Autodesk Inventor part; units mm, degrees
ref_plane "YZ Plane" through (0, 0, 0) normal (1, 0, 0) x (0, 1, 0)
ref_plane "XZ Plane" through (0, 0, 0) normal (0, 1, 0) x (-1, 0, 0)
ref_plane "XY Plane" through (0, 0, 0) normal (0, 0, 1) x (1, 0, 0)
sketch "Sketch1" plane through (0, 0, 0) normal (0, 0, 1) x (1, 0, 0)
  line L0 (0, 0) -> (26.9875, 0)
  line L1 (26.9875, 5.08) -> (0, 5.08)
  line L2 (0, 5.08) -> (0, 0)
  arc A0 (26.9875, 4.1275) -> (26.9875, 0.9525) centre (26.9875, 2.54) ccw
  line L3 (26.9875, 0) -> (26.9875, 0.9525)
  line L4 (26.9875, 4.1275) -> (26.9875, 5.08)
  dimension "d0" = 5.08
  dimension "d1" = 26.9875
  dimension "d2" = 3.175
revolve "Revolution1" add sketch "Sketch1" angle 360 about axis through (0, 5.08, 0) along (0, -1, 0)
sketch "Sketch2" plane through (0, 5.08, 0) normal (0, 1, 0) x (1, 0, 0)
  line L0 (-22.0146, 3.0506) -> (-3.175, 3.1571)
  line L1 (3.175, 3.193) -> (21.9787, 3.2993)
  line L2 (-3.175, -21.997) -> (-3.175, -3.193)
  line L3 (-3.175, 3.1571) -> (-3.175, 21.997)
  arc A0 (-3.175, 21.997) -> (-22.0146, 3.0506) centre (0, 0) ccw
  line L4 (-21.9787, -3.2993) -> (-3.175, -3.193)
  line L5 (3.175, -3.1571) -> (22.0146, -3.0506)
  arc A1 (-21.9787, -3.2993) -> (-3.175, -21.997) centre (0, 0) ccw
  line L6 (3.175, -21.997) -> (3.175, -3.1571)
  line L7 (3.175, 3.193) -> (3.175, 21.997)
  arc A2 (3.175, -21.997) -> (22.0146, -3.0506) centre (0, 0) ccw
  arc A3 (21.9787, 3.2993) -> (3.175, 21.997) centre (0, 0) ccw
extrude "Extrusion1" cut sketch "Sketch2" against normal blind 25.4
sketch "Sketch3" plane through (0, 5.08, 0) normal (0, 1, 0) x (1, 0, 0)
  arc A0 (-1.0795, -0.9837) -> (-1.0795, 0.9837) centre (0, 0) ccw
  line L0 (-1.0795, -0.9837) -> (-1.0795, 0.9837)
  dimension "d11" = 2.921
  dimension "d12" = 1.0795
extrude "Extrusion2" cut sketch "Sketch3" against normal blind 25.4
fillet "Fillet1" radius 1.585 12 edges at (-3.175, 2.54, -3.1571) (3.175, 2.54, -3.193) (3.175, 2.54, 3.1571) (-3.175, 2.54, 3.193) (-21.9787, 2.54, 3.2993) (-3.175, 2.54, 21.997) (3.175, 2.54, 21.997) (22.0146, 2.54, 3.0506) (21.9787, 2.54, -3.2993) (3.175, 2.54, -21.997) (-3.175, 2.54, -21.997) (-22.0146, 2.54, -3.0506)
chamfer "Chamfer1" distance 1.585 angle 45 48 edges at (-12.4262, 5.08, -3.1048) (-21.348, 5.08, -3.6563) (-15.7598, 5.08, -15.671) (-3.7769, 5.08, -21.3269) (-3.175, 5.08, -12.4084) (-3.6361, 5.08, -3.6156) (-12.4172, 5.08, 3.2453) (-3.6424, 5.08, 3.6631) (-3.175, 5.08, 12.4353) (-3.7769, 5.08, 21.3269) (-15.671, 5.08, 15.7598) (-21.3052, 5.08, 3.8974) (12.4262, 5.08, 3.1048) (21.348, 5.08, 3.6563) (15.7598, 5.08, 15.671) (3.7769, 5.08, 21.3269) (3.175, 5.08, 12.4084) (3.6361, 5.08, 3.6156) (12.4172, 5.08, -3.2453) (3.6424, 5.08, -3.6631) (3.175, 5.08, -12.4353) (3.7769, 5.08, -21.3269) (15.671, 5.08, -15.7598) (21.3052, 5.08, -3.8974) (-3.6361, 0, -3.6156) (-12.4262, 0, -3.1048) (-21.348, 0, -3.6563) (-15.7598, 0, -15.671) (-3.7769, 0, -21.3269) (-3.175, 0, -12.4084) (-3.175, 0, 12.4353) (-3.6424, 0, 3.6631) (-12.4172, 0, 3.2453) (-21.3052, 0, 3.8974) (-15.671, 0, 15.7598) (-3.7769, 0, 21.3269) (3.175, 0, 12.4084) (3.7769, 0, 21.3269) (15.7598, 0, 15.671) (21.348, 0, 3.6563) (12.4262, 0, 3.1048) (3.6361, 0, 3.6156) (3.175, 0, -12.4353) (3.6424, 0, -3.6631) (12.4172, 0, -3.2453) (21.3052, 0, -3.8974) (15.671, 0, -15.7598) (3.7769, 0, -21.3269)
properties part number "Wheel"
CAD build for the part. Positions are in the model's coordinates, mm. A direction names the side the tool comes from. Give positions to 0.01 mm unless a question says otherwise; leave off trailing zeros. Write each loop counter-clockwise with the first axis right and the second up, starting at its lowest first coordinate (ties: lowest second). Pieces come first, ordered by that corner, then holes. Notation, with made-up numbers: (30, 29.5) -> (83, 29.5) arc R19 ccw to (83, 41.5) -> close; hole circle Ø5 at (-8.5, 63.25). An arc over 180 degrees is marked (long way). Return JSON: item names as keys, results as strings.
Item 1: Tool access for faces 1 (the cylindrical face through (-21.3, 2.5, -3.6)), 2 (the conical face through (-3.2, 4.1, -3.2)), 3 (the conical face through (3.174, 0.958, 3.19)): list every direction of +Z, -Z, +X, -X, +Y, -Y with a clear straight run to the whole face (end or side of a thin tool).
Answer below:
{"face 1": "+Y, -Y", "face 2": "+Y", "face 3": "-Y"}
Item 2: Band-saw the part on C-C (x = 9). Give the number of separate pieces and of enclosed holes in the cut face, then the cut area to 3 significant figures.
Answer below:
{"separate pieces": "3", "enclosed holes": "0", "area": "65.4 mm2"}
Item 3: Drop flat-ended pins along their axis: pin 1 (4 mm diameter, centred on x = -4.5, z = -16.5, fed in from -Y); pin 2 (0.6 mm diameter, centred on y = 3, z = 0, fed in from +X); pin 3 (8 mm diameter, centred on x = -1, z = 2, fed in from -Y); pin 4 (1 mm diameter, centred on y = 2, z = 15.5, fed in from +X). Give the stop position or say it passes through.
Answer below:
{"pin 1": "stops at y = 0.91", "pin 2": "stops at x = 25.59", "pin 3": "stops at y = 0", "pin 4": "stops at x = 20.73"}
Item 4: Band-saw the part on A-A (z = 0). List the corners of the cut face in (x, y) (1 decimal), then the cut area to 3 significant figures.
Answer below:
{"outline": "(-27, 0) -> (-1.1, 0) -> (-1.1, 5.1) -> (-27, 5.1) -> (-27, 4.1) arc R1.6 cw to (-27, 1) -> close; (1.5, 0) -> (27, 0) -> (27, 1) arc R1.6 cw to (27, 4.1) -> (27, 5.1) -> (1.5, 5.1) -> close", "area": "253 mm2"}
Item 5: Band-saw the part on B-B (x = 0). List the corners of the cut face in (y, z) (1 decimal), then the cut area to 3 significant figures.
Answer below:
{"outline": "(0, -27) -> (1, -27) arc R1.6 cw to (4.1, -27) -> (5.1, -27) -> (5.1, -1.5) -> (0, -1.5) -> close; (0, 1.5) -> (5.1, 1.5) -> (5.1, 27) -> (4.1, 27) arc R1.6 cw to (1, 27) -> (0, 27) -> close", "area": "251 mm2"}
Item 6: Drill centre lines: probe 1 along X at (y, z) = (0.65, -7); probe 2 along X at (y, z) = (2.45, -15.5) (3 decimals); probe 3 along Y at (x, z) = (18, -20). Where is each one in solid material? Low to high.
Answer below:
{"probe 1": "x = -26.06 to -22.08, -2.24 to 2.24, 22.08 to 26.06", "probe 2": "x = -20.126 to -15.928, -3.175 to 3.175, 15.928 to 20.126", "probe 3": "y = 0 to 0.95, 4.13 to 5.08"}
